Autodesk Inventor part; units mm, degrees
ref_plane "YZ Plane" through (0, 0, 0) normal (1, 0, 0) x (0, 1, 0)
ref_plane "XZ Plane" through (0, 0, 0) normal (0, 1, 0) x (-1, 0, 0)
ref_plane "XY Plane" through (0, 0, 0) normal (0, 0, 1) x (1, 0, 0)
sketch "Эскиз1" plane through (0, 0, 0) normal (0, 0, 1) x (1, 0, 0)
  line L0 (7.5, -5) -> (7.5, 0)
  line L1 (5.0577, -5) -> (7.5, -5)
  line L2 (5.0577, -5) -> (-4.3392, -5)
  line L3 (-6.7815, -5) -> (-4.3392, -5)
  line L4 (-6.7815, -5) -> (-6.7815, 0)
  line L5 (-6.7815, 0) -> (-4.3392, 0)
  line L6 (5.0577, 0) -> (-4.3392, 0)
  line L7 (5.0577, 0) -> (7.5, 0)
  line L8 (7.5, -10.5) -> (-7.5, -10.5)
  line L9 (7.5, 0) -> (-6.7815, 0)
  line L10 (7.5, 10.5) -> (7.5, 0)
  line L11 (-7.5, 10.5) -> (7.5, 10.5)
  line L12 (-7.5, -10.5) -> (-7.5, 10.5)
  line L13 (7.5, -10.5) -> (-7.5, -10.5)
  line L14 (7.5, -5) -> (7.5, -10.5)
  line L15 (7.5, -5) -> (-6.7815, -5)
  line L16 (-6.7815, -5) -> (-6.7815, 0)
  point P0 (0, 0)
extrude "Выдавливание1" add sketch "Эскиз1" along normal blind 10 contours L14 L8 L12 L11 L10 L7 L6 L5 L4 L3 L2 L1
sketch "Эскиз2" plane through (-7.5, 10.5, 0) normal (0, 1, 0) x (1, 0, 0)
  circle A0 centre (7.8593, -5) radius 2
  point P0 (7.5, 0)
extrude "Выдавливание2" cut sketch "Эскиз2" against normal through all
sketch "Эскиз3" plane through (-7.5, 10.5, 0) normal (0, 1, 0) x (1, 0, 0)
  line L0 (15, -10) -> (0, -10)
  line L1 (15, -10) -> (15, -15.4596)
  line L2 (15, -15.4596) -> (0, -10)
  point P0 (7.5, 0)
  dimension "d5" = 20
extrude "Выдавливание3" add sketch "Эскиз3" against normal up to surface (21 mm away)
sketch "Эскиз4" plane through (7.5, -10.5, 15.4596) normal (-0.3420201, 0, 0.9396926) x (0.9396926, 0, 0.3420201)
  line L0 (-15.9627, 0) -> (0, 0)
  line L1 (0, 21) -> (0, 0)
  line L2 (-15.9627, 21) -> (0, 21)
  line L3 (-15.9627, 21) -> (-15.9627, 0)
  line L4 (-17.9813, -2.0187) -> (2.0187, -2.0187)
  line L5 (2.0187, -2.0187) -> (2.0187, 23.0187)
  line L6 (2.0187, 23.0187) -> (-17.9813, 23.0187)
  line L7 (-17.9813, 23.0187) -> (-17.9813, -2.0187)
  point P0 (-12.3352, 10.5)
  dimension "d8" = 20
extrude "Выдавливание4" add sketch "Эскиз4" along normal blind 2 contours L3 L2 L1 L0 | L7 L6 L5 L4
sketch "Эскиз5" plane through (6.816, -10.5, 17.3389) normal (-0.3420201, 0, 0.9396926) x (0.9396926, 0, 0.3420201)
  line L0 (0.5187, 19) -> (-16.4813, 19)
  line L1 (-16.4813, 19) -> (-16.4813, 2)
  line L2 (-16.4813, 2) -> (0.5187, 2)
  line L3 (0.5187, 2) -> (0.5187, 19)
  line L4 (2.0187, -2.0187) -> (2.0187, 23.0187)
  line L5 (-17.9813, -2.0187) -> (2.0187, -2.0187)
  line L6 (-0.4813, 18) -> (-15.4813, 18)
  line L7 (-15.4813, 18) -> (-15.4813, 3)
  line L8 (-15.4813, 3) -> (-0.4813, 3)
  line L9 (-0.4813, 3) -> (-0.4813, 18)
  point P0 (-12.3352, 10.5)
  point P1 (0.5187, 10.5)
  point P2 (2.0187, 10.5)
  point P3 (-7.9813, 2)
  point P4 (-7.9813, -2.0187)
  dimension "d11" = 17
  dimension "d12" = 1
extrude "Выдавливание5" add sketch "Эскиз5" along normal blind 8
fillet "Сопряжение1" radius 2 8 edges at (5.9353, -8.5, 21.2751) (5.9353, 8.5, 21.2751) (-10.0395, 8.5, 15.4608) (-10.0395, -8.5, 15.4608) (-9.0998, 7.5, 15.8028) (4.9956, 7.5, 20.9331) (-9.0998, -7.5, 15.8028) (4.9956, -7.5, 20.9331)
equation "\"degg\" = 70deg"
properties part number "base_70"
Work out the finished part from the listing and answer in its coordinate system (mm). A direction names the side the tool comes from. Round coordinates to 2 decimals unless told otherwise and drop trailing zeros. Write each loop counter-clockwise with the first axis right and the second up, starting at its lowest first coordinate (ties: lowest second). Pieces come first, ordered by that corner, then holes.
1) A cutting plane is placed at C-C (x = -2). Give the vertices of the cut face in (y, z).
2) Straight lines are drawn through the part: line 1 (Y direction, x = -0.75, z = 17.25); line 2 (Y direction, x = -2.75, z = 4.5); line 3 (X direction, y = 4.5, z = 5). For each, find the intervals that lie inside material, in ascending order.
3) A tool of negligible diameter and unlimited length cuts with its end or side. For faces 1 (the flat face through (0, -2, 10)), 2 (the flat face through (-9.17, 2.96, 11.52)), 3 (the flat face through (7.5, 2, 8)), 4 (the cylindrical face through (-9.52, -7.9, 15.71)), 5 (the flat face through (-10.02, 0.09, 15.41)), from which of +Z, -Z, +X, -X, +Y, -Y can it reach the whole face along a straight path? Write none if from no direction.
4) The mould has two halves that part along Y. Classify faces 6 (the flat face through (8.22, 0.18, 15.72)), 7 (the flat face through (5.015, -0.077, 20.88)), 8 (the flat face through (0, -10.5, 8)): pulls with the +Y half, pulls with the -Y half, needs draft (parallel to the pull), parting line crosses it, or undercut.
5) Given pin 1 Ø11 at (y, z) = (-2, 6) entering from -X; pin 2 Ø3 at (x, z) = (-1, 4.5) entering from -Y; pin 3 Ø5.5 at (x, z) = (-2.5, 21) entering from -Y, each flat-ended and moving along its own axis, determine where each tip first touches the part or whether it passes through.
6) A cutting plane is placed at A-A (z = 5). Give the vertices of the cut face in (x, y), plus the area to 3 significant figures.
7) A cutting plane is placed at D-D (y = -1). Give the vertices of the cut face in (x, z), plus the area to 3 significant figures.
8) A cutting plane is placed at B-B (y = 2.75). Give the vertices of the cut face in (x, z), plus the area to 3 significant figures.
Completed:
1. outline: (-12.52, 12) - (-10.5, 12) - (-10.5, 0) - (-5, 0) - (-5, 10) - (0, 10) - (0, 0) - (10.5, 0) - (10.5, 12) - (12.52, 12) - (12.52, 14.13) - (8.5, 14.13) - (8.5, 22.64) - (7.5, 22.64) - (7.5, 14.13) - (-7.5, 14.13) - (-7.5, 22.64) - (-8.5, 22.64) - (-8.5, 14.13) - (-12.52, 14.13) - close
2. line 1: y = -8.5 to -7.5, 7.5 to 8.5
2. line 2: y = -10.5 to -5, 0 to 10.5
2. line 3: x = -7.5 to -1.64, 2.36 to 7.5
3. face 1: -Z, +X
3. face 2: none
3. face 3: -Z, +X, +Y, -Y
3. face 4: -X, -Y
3. face 5: -X, +Y, -Y
4. face 6: needs draft
4. face 7: undercut
4. face 8: pulls with the -Y half
5. pin 1: stops at x = -10.08
5. pin 2: stops at y = -10.5
5. pin 3: stops at y = -8.5
6. outline: (-7.5, -10.5) - (-1.64, -10.5) - (-1.64, -5) - (-6.78, -5) - (-6.78, 0) - (-1.64, 0) - (-1.64, 10.5) - (-7.5, 10.5) - close; (2.36, -10.5) - (7.5, -10.5) - (7.5, -5) - (2.36, -5) - close; (2.36, 0) - (7.5, 0) - (7.5, 10.5) - (2.36, 10.5) - close
6. area: 180 mm2
7. outline: (-11.41, 19.22) - (-8.67, 11.7) - (-10.08, 11.19) - (-9.4, 9.31) - (-7.5, 10) - (-7.5, 0) - (-6.78, 0) - (-6.78, 10) - (7.5, 10) - (7.5, 15.46) - (9.4, 16.15) - (8.71, 18.03) - (7.3, 17.52) - (4.57, 25.03) - (3.63, 24.69) - (6.36, 17.17) - (-7.73, 12.04) - (-10.47, 19.56) - close
7. area: 104 mm2
8. outline: (-11.41, 19.22) - (-8.67, 11.7) - (-10.08, 11.19) - (-9.4, 9.31) - (-7.5, 10) - (-7.5, 0) - (7.5, 0) - (7.5, 15.46) - (9.4, 16.15) - (8.71, 18.03) - (7.3, 17.52) - (4.57, 25.03) - (3.63, 24.69) - (6.36, 17.17) - (-7.73, 12.04) - (-10.47, 19.56) - close; hole circle Ø4 at (0.36, 5)
8. area: 234 mm2
